Check sheet for the drawn part. Datum: minimum x, y, z corner. Units: mm. A direction names the side the tool comes from. Round coordinates to 2 decimals unless told otherwise and drop trailing zeros. Write each loop counter-clockwise with the first axis right and the second up, starting at its lowest first coordinate (ties: lowest second). Pieces come first, ordered by that corner, then holes. Notation, with made-up numbers: M 26,-35 L 83,-35 A5 ccw 83,-26 Z; hole C 17.5,77 d11. An arc over 180 degrees is marked long. One line per item, written item: value. Start each with the question number.
1. Depth check by flat-ended pin: P1, Ø3, axis at x = 3.5, z = 22.5, coming from the +Y side; P2, Ø0.6, axis at y = 11.5, z = 3, coming from the -X side; P3, Ø2, axis at y = 12, z = 7.5, coming from the +X side. Enter the tip coordinate at first touch or a pass-through.
2. Section check B-B (y = 11.5). Record the boundary of the cut face in (x, z), and give its area (3 significant figures).
3. Scan lines: probe 1 along Y at (x, z) = (6, 6.5); probe 2 along Z at (x, y) = (0.5, 6); probe 3 along Z at (x, y) = (2.25, 2.5). Record each from-to range of solid material in increasing order. Write a range as [from, to].
4. Section check A-A (z = 7.5). Record the boundary of the cut face in (x, y).
5. Access from +Z, -Z, +X, -X, +Y, -Y to the whole of each face (thin tool, end or side, straight path). Record for the marked faces 1, 2 and 3.
6. Section check D-D (y = 7). Record the boundary of the cut face in (x, z), and give its area (3 significant figures).
7. Section check C-C (x = 3.75). Record the boundary of the cut face in (y, z).
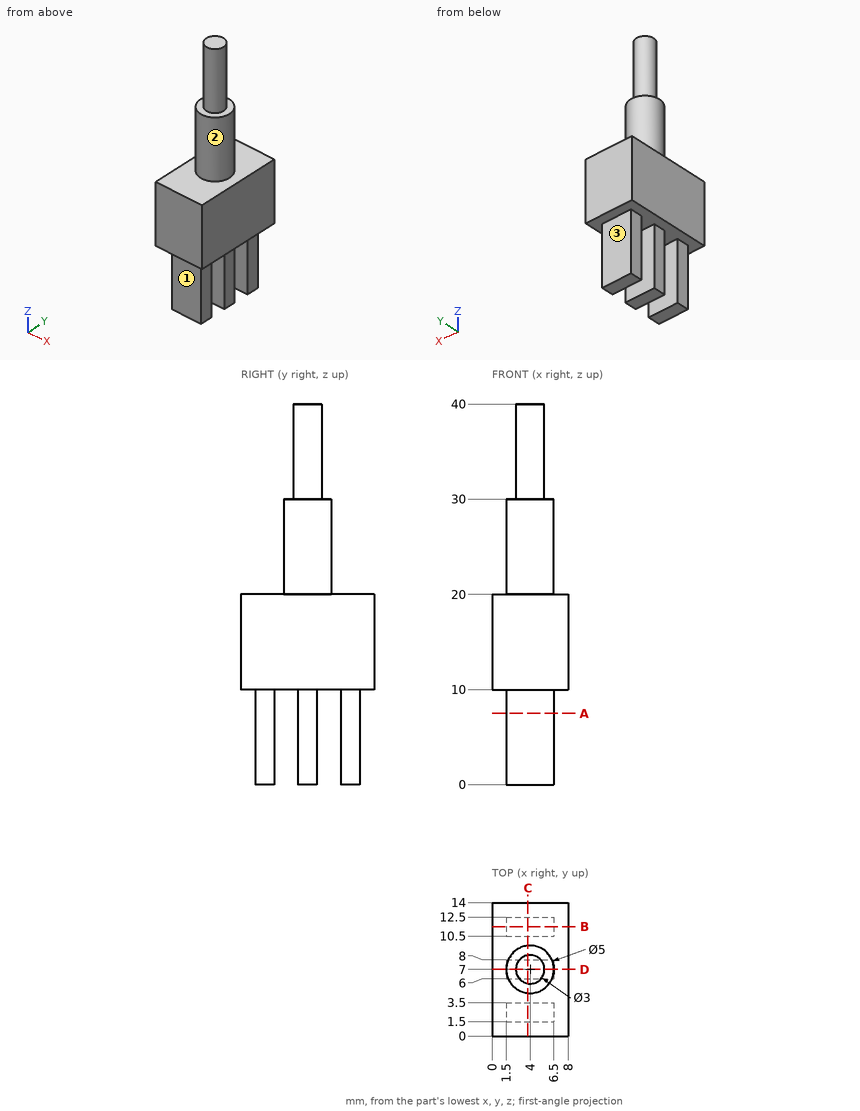
Result sheet:
1. P1: stops at y = 9.5
1. P2: stops at x = 1.5
1. P3: stops at x = 6.5
2. outline: M 0,10 L 1.5,10 L 1.5,0 L 6.5,0 L 6.5,10 L 8,10 L 8,20 L 0,20 Z
2. area: 130 mm2
3. probe 1: y = [1.5, 3.5], [6, 8], [10.5, 12.5]
3. probe 2: z = [10, 20]
3. probe 3: z = [0, 20]
4. outline: M 1.5,1.5 L 6.5,1.5 L 6.5,3.5 L 1.5,3.5 Z; M 1.5,6 L 6.5,6 L 6.5,8 L 1.5,8 Z; M 1.5,10.5 L 6.5,10.5 L 6.5,12.5 L 1.5,12.5 Z
5. face 1: -Z, +X, -X, -Y
5. face 2: +Z
5. face 3: -Z, +X, -X, +Y
6. outline: M 0,10 L 1.5,10 L 1.5,0 L 6.5,0 L 6.5,10 L 8,10 L 8,20 L 6.5,20 L 6.5,30 L 5.5,30 L 5.5,40 L 2.5,40 L 2.5,30 L 1.5,30 L 1.5,20 L 0,20 Z
6. area: 210 mm2
7. outline: M 0,10 L 1.5,10 L 1.5,0 L 3.5,0 L 3.5,10 L 6,10 L 6,0 L 8,0 L 8,10 L 10.5,10 L 10.5,0 L 12.5,0 L 12.5,10 L 14,10 L 14,20 L 9.49,20 L 9.49,30 L 8.48,30 L 8.48,40 L 5.52,40 L 5.52,30 L 4.51,30 L 4.51,20 L 0,20 Z
